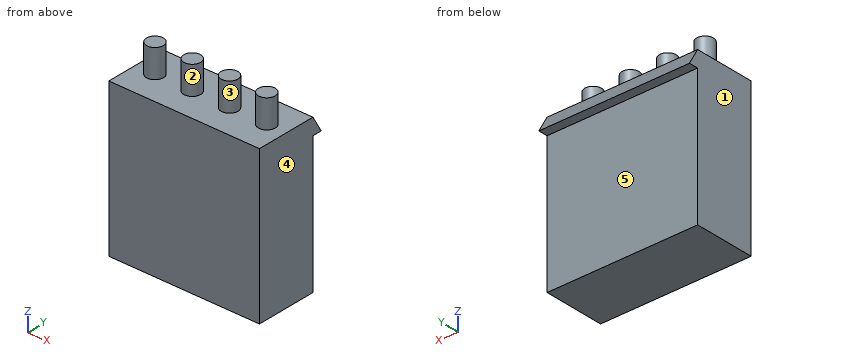
Autodesk Inventor part; units mm, degrees
ref_plane "YZ Plane" through (0, 0, 0) normal (1, 0, 0) x (0, 1, 0)
ref_plane "XZ Plane" through (0, 0, 0) normal (0, 1, 0) x (-1, 0, 0)
ref_plane "XY Plane" through (0, 0, 0) normal (0, 0, 1) x (1, 0, 0)
sketch "Boceto1" plane through (0, 0, 0) normal (0, 1, 0) x (-1, 0, 0)
  line L0 (8, 8.175) -> (-8, 8.175)
  line L1 (-8, 8.175) -> (-8, -8.175)
  line L2 (-8, -8.175) -> (8, -8.175)
  line L3 (8, -8.175) -> (8, 8.175)
  point P0 (0, 0)
  dimension "d0" = 16.35
  dimension "d1" = 16
  dimension "d2" = 8
  dimension "d3" = 8.175
extrude "Extrusión1" add sketch "Boceto1" along normal mid plane 6.5
sketch "Boceto2" plane through (8, -3.25, -8.175) normal (1, 0, 0) x (0, 0, -1)
  line L0 (0, 0) -> (0, 6.5)
  line L1 (-16.35, 6.5) -> (0, 6.5)
  line L2 (-16.35, 0) -> (-16.35, 6.5)
  line L3 (0, 0) -> (-16.35, 0)
  line L4 (0, 6.5) -> (-16.35, 6.5)
  line L5 (-16.35, 6.5) -> (-14.6179, 7.5)
  line L6 (-14.6179, 7.5) -> (-14.6179, 6.5)
  line L7 (-16.35, 6.5) -> (-14.6179, 6.5)
  point P0 (-8.175, 3.25)
  dimension "d6" = 7.5
  dimension "d7" = 60
extrude "Extrusión2" add sketch "Boceto2" against normal blind 16 contours L1 L5 L6
sketch "Boceto3" plane through (-8, -3.25, 8.175) normal (0, 0, 1) x (1, 0, 0)
  line L0 (16, 0) -> (16, 6.5)
  line L1 (0, 6.5) -> (16, 6.5)
  line L2 (0, 0) -> (0, 6.5)
  line L3 (16, 0) -> (0, 0)
  circle A0 centre (13.94, 3.25) radius 0.9
  circle A1 centre (9.98, 3.25) radius 0.9
  circle A2 centre (6.02, 3.25) radius 0.9
  circle A3 centre (2.06, 3.25) radius 0.9
  point P0 (8, 3.25)
  dimension "d10" = 3.25
  dimension "P" = 3.96
  dimension "d12" = 3.96
  dimension "d13" = 3.96
  dimension "d14" = 2.06
  dimension "d15" = 1.8
  dimension "d16" = 1.8
  dimension "d17" = 1.8
  dimension "d18" = 1.8
extrude "Extrusión3" add sketch "Boceto3" along normal blind 3 contours A0 | A1 | A2 | A3
properties part number "conector_4pines"
Work out the finished part from the listing and answer in its coordinate system (mm). Face numbers are marked on the shaded views. A direction names the side the tool comes from. Round coordinates to 2 decimals unless told otherwise and drop trailing zeros. Order: outer loops, then holes, each group sorted by start corner. A loop starts at its lowest first (then second) coordinate and runs counter-clockwise, first axis right, second up. Notation, with made-up numbers: M 24,49.5 L 77,49.5 A35 ccw 77,88.5 Z; hole C 45,-18 d3. An arc over 180 degrees is marked long. Put each result on its own line as item: value. Start each with the question number.
Q1. Section A-A, the plane x = 5.94 is taken. Write down the section's boundary in (y, z) (3 decimals).
Q2. Straight lines are drawn through the part: L1, parallel to Z at x = 5.75, y = -1.5 (3 decimals); L2, parallel to Y at x = -2.5, z = 4.75; L3, parallel to Z at x = 4, y = 4. For each, find the intervals that lie inside material, in ascending order. Write a range as [from, to].
Q3. For a pull along X with two mould halves and no side action, classify the marked faces 3, 4 and 5 as pulls with the +X half, pulls with the -X half, needs draft (parallel to the pull), parting line crosses it, or undercut.
Q4. Section C-C, the plane z = 1.75 is taken. Write down the section's boundary in (x, y), and give its area (3 significant figures).
Q5. Section B-B, the plane y = 0 is taken. Write down the section's boundary in (x, z) (3 decimals).
Q6. Flat-ended cylindrical pins translate along their axes: pin 1 (0.8 mm diameter, centred on x = 0, y = 4, fed in from -Z); pin 2 (6 mm diameter, centred on x = 2, z = 5.5, fed in from +Y); pin 3 (7.5 mm diameter, centred on x = 4, z = 2.5, fed in from +Y). Find the tip coordinate at first contact, or state that the pin passes through.
Q7. A tool of negligible diameter and unlimited length cuts with its end or side. For the marked faces 1 and 2, from which of +Z, -Z, +X, -X, +Y, -Y can it reach the whole face along a straight path? Write none if from no direction.
Q8. Section D-D, the plane x = -0.75 is taken. Write down the section's boundary in (y, z) (3 decimals), and give its area (3 significant figures).
Findings below:
1. outline: M -3.25,-8.175 L 3.25,-8.175 L 3.25,6.443 L 4.25,6.443 L 3.25,8.175 L 0.9,8.175 L 0.9,11.175 L -0.9,11.175 L -0.9,8.175 L -3.25,8.175 Z
2. L1: z = [-8.175, 8.175]
2. L2: y = [-3.25, 3.25]
2. L3: z = [6.44, 6.88]
3. face 3: undercut
3. face 4: pulls with the +X half
3. face 5: needs draft
4. outline: M -8,-3.25 L 8,-3.25 L 8,3.25 L -8,3.25 Z
4. area: 104 mm^2
5. outline: M -8,-8.175 L 8,-8.175 L 8,8.175 L 6.84,8.175 L 6.84,11.175 L 5.04,11.175 L 5.04,8.175 L 2.88,8.175 L 2.88,11.175 L 1.08,11.175 L 1.08,8.175 L -1.08,8.175 L -1.08,11.175 L -2.88,11.175 L -2.88,8.175 L -5.04,8.175 L -5.04,11.175 L -6.84,11.175 L -6.84,8.175 L -8,8.175 Z
6. pin 1: stops at z = 6.44
6. pin 2: stops at y = 4.25
6. pin 3: stops at y = 3.25
7. face 1: +Z, -Z, -X, +Y, -Y
7. face 2: +Z
8. outline: M -3.25,-8.175 L 3.25,-8.175 L 3.25,6.443 L 4.25,6.443 L 3.25,8.175 L -3.25,8.175 Z
8. area: 107 mm^2
